Geometry check sheet. Reference: drawing and pictorial views, mm from the part's lowest x, y, z. A direction names the side the tool comes from. Give positions to 0.01 mm unless a question says otherwise; leave off trailing zeros. Write each loop counter-clockwise with the first axis right and the second up, starting at its lowest first coordinate (ties: lowest second). Pieces come first, ordered by that corner, then holes. Notation, with made-up numbers: (-8.75, 7.5) -> (29.25, 7.5) arc R25 cw to (29.25, 32.5) -> close; hole circle Ø3 at (87, 63). An arc over 180 degrees is marked (long way). Return JSON: item names as keys, results as strings.
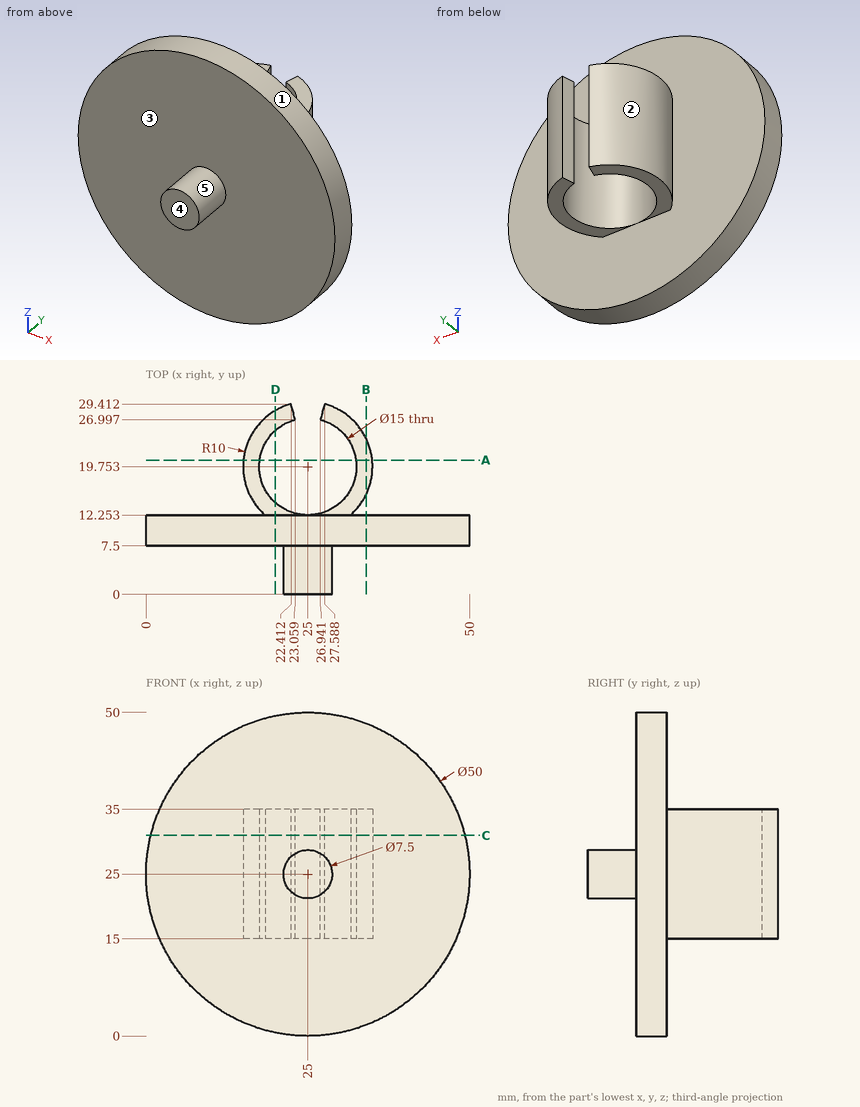
(1) Release check for a two-part mould opening along Y. For the marked faces 1, 2 and 3 record: pulls with the +Y half, pulls with the -Y half, needs draft (parallel to the pull), parting line crosses it, or undercut.
Reply:
{"face 1": "needs draft", "face 2": "undercut", "face 3": "pulls with the -Y half"}
(2) Thickness scan on L1, parallel to Y at x = 41, z = 9; L2, parallel to X at y = 15.5, z = 29; L3, parallel to X at y = 20.25, z = 23.5. Record the ranges inside material, lowest first.
Reply:
{"L1": "7.5 to 12.25", "L2": "15.95 to 18.82, 31.18 to 34.05", "L3": "15.01 to 17.52, 32.48 to 34.99"}
(3) Set-up check for the marked faces 4 and 5: record each of +Z, -Z, +X, -X, +Y, -Y from which the full face is reachable in a straight line by a thin tool's end or side.
Reply:
{"face 4": "+Z, -Z, +X, -X, -Y", "face 5": "-Y"}
(4) Cross-section at C-C on z = 31. Enter the section's corners in (x, y), then the cut area to 3 significant figures.
Reply:
{"outline": "(0.73, 7.5) -> (49.27, 7.5) -> (49.27, 12.25) -> (31.61, 12.25) arc R10 ccw to (27.59, 29.41) -> (26.94, 27) arc R7.5 cw (long way) to (23.06, 27) -> (22.41, 29.41) arc R10 ccw to (18.39, 12.25) -> (0.73, 12.25) -> close", "area": "334 mm^2"}
(5) Cross-section at B-B on x = 34. Enter the section's corners in (y, z), then the cut area to 3 significant figures.
Reply:
{"outline": "(7.5, 1.68) -> (12.25, 1.68) -> (12.25, 48.32) -> (7.5, 48.32) -> close; (15.39, 15) -> (24.11, 15) -> (24.11, 35) -> (15.39, 35) -> close", "area": "396 mm^2"}
(6) Cross-section at D-D on x = 20. Enter the section's corners in (y, z) (1 decimal).
Reply:
{"outline": "(7.5, 0.5) -> (12.3, 0.5) -> (12.3, 15) -> (14.2, 15) -> (14.2, 35) -> (12.3, 35) -> (12.3, 49.5) -> (7.5, 49.5) -> close; (25.3, 15) -> (28.4, 15) -> (28.4, 35) -> (25.3, 35) -> close"}
(7) Cross-section at A-A on y = 20.75. Enter the section's corners in (x, z), then the cut area to 3 significant figures.
Reply:
{"outline": "(15.05, 15) -> (17.57, 15) -> (17.57, 35) -> (15.05, 35) -> close; (32.43, 15) -> (34.95, 15) -> (34.95, 35) -> (32.43, 35) -> close", "area": "101 mm^2"}
(8) Depth check by flat-ended pin: pin 1 Ø5 at (x, y) = (18.5, 24) entering from +Z; pin 2 Ø4 at (x, y) = (34.5, 25.5) entering from -Z; pin 3 Ø1 at (x, y) = (28, 14) entering from -Z; pin 4 Ø8 at (x, y) = (40, 15.5) entering from -Z (1 decimal). Enter the tip coordinate at first touch or a pass-through.
Reply:
{"pin 1": "z = 35", "pin 2": "z = 15", "pin 3": "through", "pin 4": "z = 3.4"}
